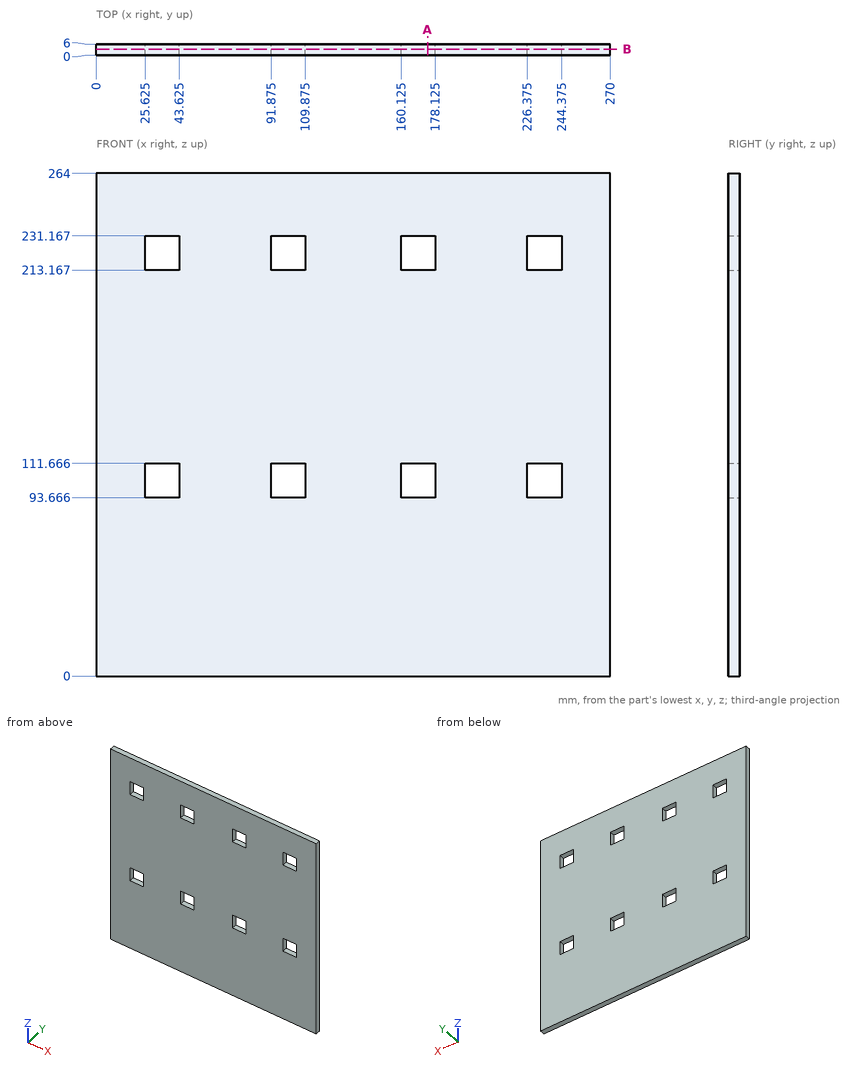
Answer from the drawing. Dimensions are ordinates in mm from the lowest x, y and z of the part. Give positions to 0.01 mm unless a question says otherwise; leave off trailing zeros. Write each loop counter-clockwise with the first axis right and the second up, starting at its lowest first coordinate (ties: lowest second). Pieces come first, ordered by that corner, then holes. Notation, with made-up numbers: M 45.25,32.5 L 84.25,32.5 A23 cw 84.25,48.5 Z; hole C -8,26.5 d5. An arc over 180 degrees is marked long. Answer as CSV lines item,"result".
Q1. A cutting plane is placed at A-A on x = 174. Write down the section's boundary in (y, z).
A:
outline,"M 0,0 L 6,0 L 6,93.67 L 0,93.67 Z; M 0,111.67 L 6,111.67 L 6,213.17 L 0,213.17 Z; M 0,231.17 L 6,231.17 L 6,264 L 0,264 Z"
Q2. Find the intervals of material crossed by probe 1 along Z at (x, y) = (42, 1.1); probe 2 along X at (y, z) = (2.7, 104.5) (1 decimal), in increasing order. Write a range as [from, to].
A:
probe 1,"z = [0, 93.67], [111.67, 213.17], [231.17, 264]"
probe 2,"x = [0, 25.6], [43.6, 91.9], [109.9, 160.1], [178.1, 226.4], [244.4, 270]"
Q3. A cutting plane is placed at B-B on y = 3.35. Count the separate pieces of the cut face and the enclosed holes in it, plus the area to 3 significant figures.
A:
separate pieces,"1"
enclosed holes,"8"
area,"68,700 mm²"
